```python
from build123d import *

# Parameters (mm, degrees)
ESQUISSE1_R                      = 1.7
BOSS_EXTRU_1_DEPTH               = 4.5
CONG_1_R                         = 3
R_P_TITION_START                 = 3
R_P_TITION_CIRCULAIRE1_OUTLINE_R = 1.7
R_P_TITION_CIRCULAIRE1_DEPTH     = 4.5
CHANFREIN1_SIZE                  = 1.05


# Read off the part's stored shape, not the designer's step: Répétition circulaire1
with BuildPart() as part:
    # Sketch1 → Revolve1 (revolve)
    with BuildSketch(Plane.XY, mode=Mode.PRIVATE) as revolve1_sk:
        Polygon((9, 0), (27, 0), (27, 3), (29, 3), (29, 7.5), (6.5, 7.5), (6.5, 6), (8, 6), (8, 1), align=None)
    revolve(revolve1_sk.sketch.rotate(Axis((0, 16.318563478, 0), (0, -1, 0)), 90), axis=Axis((0, 16.318563478, 0), (0, -1, 0)))

    # Esquisse1 → Boss.-Extru.1 (add)
    with BuildSketch(Plane(origin=(0, 7.5, 0), x_dir=(1, 0, 0), z_dir=(0, 1, 0))):
        with BuildLine():
            Line((-4.5, 33), (-4.5, 28.648734702))
            ThreePointArc((-4.5, 28.648734702), (0, 29), (4.5, 28.648734702))
            Line((4.5, 28.648734702), (4.5, 33))
            ThreePointArc((4.5, 33), (0, 37.5), (-4.5, 33))
        make_face()
        with Locations(Location((0, 33, 0), (0, 0, 270))):
            Circle(ESQUISSE1_R, mode=Mode.SUBTRACT)
    extrude(amount=-BOSS_EXTRU_1_DEPTH)

    # Congé1
    cong_1_edges = [part.edges().sort_by_distance(p)[0] for p in [
        (-4.5, 5.25, -28.648734702),
        (4.5, 5.25, -28.648734702),
    ]]
    fillet(cong_1_edges, radius=CONG_1_R)

    # Répétition circulaire1 outline → Répétition circulaire1 (add)
    # profile 1 of 2: a face of its own
    with BuildSketch(Plane(origin=(0, 0, 0), x_dir=(1, 0, 0), z_dir=(0, 1, 0)).offset(R_P_TITION_START)):
        with BuildLine():
            ThreePointArc((26.328838325, -20.397114317), (32.475952642, -18.75), (30.828838325, -12.602885683))
            Line((30.828838325, -12.602885683), (29.190907557, -11.657225913))
            ThreePointArc((29.190907557, -11.657225913), (27.905010686, -10.172154026), (27.813634974, -8.209854417))
            ThreePointArc((27.813634974, -8.209854417), (25.11473671, -14.5), (21.016759974, -19.98238725))
            ThreePointArc((21.016759974, -19.98238725), (22.761849141, -19.080371134), (24.690907557, -19.451454547))
            Line((24.690907557, -19.451454547), (26.328838325, -20.397114317))
        make_face()
        with Locations((28.578838325, -16.5)):
            Circle(R_P_TITION_CIRCULAIRE1_OUTLINE_R, mode=Mode.SUBTRACT)
    # profile 2 of 2: a face of its own
    with BuildSketch(Plane(origin=(0, 0, 0), x_dir=(1, 0, 0), z_dir=(0, 1, 0)).offset(R_P_TITION_START)):
        with BuildLine():
            ThreePointArc((-20.938087556, -23.443474348), (-19.10277383, -22.743051047), (-17.227563034, -23.328331957))
            ThreePointArc((-17.227563034, -23.328331957), (-22.21528885, -18.640840681), (-25.965457103, -12.914915309))
            ThreePointArc((-25.965457103, -12.914915309), (-25.714694862, -14.863270403), (-26.723176043, -16.54907436))
            Line((-26.723176043, -16.54907436), (-28.172010867, -17.764791126))
            ThreePointArc((-28.172010867, -17.764791126), (-28.726666617, -24.104535364), (-22.386922379, -24.659191114))
            Line((-22.386922379, -24.659191114), (-20.938087556, -23.443474348))
        make_face()
        with Locations((-25.279466623, -21.21199112)):
            Circle(R_P_TITION_CIRCULAIRE1_OUTLINE_R, mode=Mode.SUBTRACT)
    extrude(amount=R_P_TITION_CIRCULAIRE1_DEPTH)

    # Chanfrein1
    chanfrein1_edges = [part.edges().sort_by_distance(p)[0] for p in [
        (0, 7.5, -34.7),
        (26.878838325, 7.5, 16.5),
        (-26.979466623, 7.5, 21.21199112),
    ]]
    chamfer(chanfrein1_edges, length=CHANFREIN1_SIZE)


solid = part.part
```
The listing builds one solid part. Answer for the finished solid, in the listing's coordinates (mm). A direction names the side the tool comes from. Coordinates: 2 decimals unless noted, no trailing zeros. Loops run counter-clockwise (first coordinate to the right, second up) from the corner with the lowest first, then second, coordinate; pieces in that order, holes last. Notation, with made-up numbers: M -22,-10 L 19,-10 A24 cw 19,7 Z; hole C -2,-13 d1. An arc over 180 degrees is marked long. Answer as CSV lines item,"result". Start each with the question number.
(1) The part is cut by section B-B (x = 0). Give the vertices of the cut face in (y, z).
(2) The part is cut by section D-D (x = 10). Give the vertices of the cut face in (y, z).
(3) Given pin 1 (0.9 mm diameter, centred on y = 5.5, z = -31.5, fed in from +X); pin 2 (2 mm diameter, centred on y = 3.5, z = -4.5, fed in from +X); pin 3 (13 mm diameter, centred on x = -0.5, z = -0.5, fed in from -Y), each flat-ended and moving along its own axis, determine where each tip first touches the part or whether it passes through.
(4) The part is cut by section A-A (z = 0). Give the vertices of the cut face in (x, y), and give its area (4 significant figures).
(5) The part is cut by section C-C (y = 2). Give the vertices of the cut face in (x, z), and give its area (3 significant figures).
(6) For faces 4 (the cylindrical face through (7.81, 3.46, -1.73)), 5 (the flat face through (-4.5, 5, -32)), 6 (the flat face through (-27.44, 5.22, 17.15)), determine the directions among +Z, -Z, +X, -X, +Y, -Y from which every point of the face is accessible in a straight line to the end or side of a thin tool.
(7) The mould has two halves that part along X. Classify faces 1 (the cylindrical face through (0.1, 5.3, -37.5)), 2 (the cylindrical face through (27.916, 5.219, 10.198)), 3 (the cylindrical face through (3.955, 6.74, -5.158)): pulls with the +X half, pulls with the -X half, needs draft (parallel to the pull), parting line crosses it, or undercut.
(8) Find the intervals of material crossed by L1, parallel to X at y = 4.55, z = -33; L2, parallel to X at y = 4.95, z = 0; L3, parallel to Y at x = 27.5, z = -1, in increasing order. Write a range as [from, to].
Determined:
1,outline,"M 0,-27 L 3,-27 L 3,-31.3 L 6.45,-31.3 L 7.5,-30.25 L 7.5,-6.5 L 6,-6.5 L 6,-8 L 1,-8 L 0,-9 Z; M 0,9 L 1,8 L 6,8 L 6,6.5 L 7.5,6.5 L 7.5,29 L 3,29 L 3,27 L 0,27 Z; M 3,-37.5 L 7.5,-37.5 L 7.5,-35.75 L 6.45,-34.7 L 3,-34.7 Z"
2,outline,"M 0,-25.08 L 3,-25.08 L 3,-27.22 L 7.5,-27.22 L 7.5,27.22 L 3,27.22 L 3,25.08 L 0,25.08 Z"
3,pin 1,"x = 4.5"
3,pin 2,"x = 28.79"
3,pin 3,"y = 6"
4,outline,"M -29,3 L -27,3 L -27,0 L -9,0 L -8,1 L -8,6 L -6.5,6 L -6.5,7.5 L -29,7.5 Z; M 6.5,6 L 8,6 L 8,1 L 9,0 L 27,0 L 27,3 L 29,3 L 29,7.5 L 6.5,7.5 Z"
4,area,"306.5 mm2"
5,outline,"C 0,0 d54; hole C 0,0 d16"
5,area,"2,090 mm2"
6,face 4,"-Y"
6,face 5,"-Z, -X, +Y, -Y"
6,face 6,"-X, +Y, -Y"
7,face 1,"parting line crosses it"
7,face 2,"pulls with the +X half"
7,face 3,"undercut"
8,L1,"[-4.5, -1.7], [1.7, 4.5]"
8,L2,"[-29, -8], [8, 29]"
8,L3,"[3, 7.5]"
